from build123d import *

# Parameters (mm, degrees)
F4_DEPTH    = 13
F5_R        = 7
F6_DEPTH    = 15
F7_R        = 14.5
F8_DEPTH    = 1.6
F9_S5_R     = 14.5
F9_T6_DEPTH = 29
F10_SIZE    = 5


# Not quite as in the source:
# - a fillet or chamfer that OpenCascade refuses, or shapes differently, is made with other operations: its cross-section is extruded or revolved along the edge and cut away or added
# - a feature names something its author has since deleted; it is built from what else it names


with BuildPart() as f2:
    # F0 (on Front) → F2 (revolve)
    with BuildSketch(Plane.XZ):
        Polygon((17.6, 24.4003517207), (0, 24.4003517207), (0, 23.0003517207), (14, 23.0003517207), (33.795146799, -22.8053483963), (43.2849223453, -22.5459427606), (43.2849223453, -21.1459427606), (37.9849223453, -21.1459427606), align=None)
    revolve(axis=Axis((0, 0, 12.0206931606), (0, 0, -1)))

    # F3 (on face) → F4 (join)
    with BuildSketch(Plane.XY.offset(24.4003517207)):
        Polygon((-11.9566419536, 1.0191727989), (-6.8609505115, -9.8451692763), (5.0956914421, -10.8643420752), (11.9566419536, -1.0191727989), (6.8609505115, 9.8451692763), (-5.0956914421, 10.8643420752), align=None)
    extrude(amount=F4_DEPTH)

    # F5 (on face) → F6 (cut)
    with BuildSketch(Plane.XY.offset(37.4003517207)):
        Circle(F5_R)
    extrude(amount=-F6_DEPTH, mode=Mode.SUBTRACT)

    # F7 (on face) → F8 (join)
    with BuildSketch(Plane.XY.offset(24.4003517207)):
        Circle(F7_R)
    extrude(amount=F8_DEPTH)

    # F9: chamfer of 4 on 1 edges, made by hand


with BuildPart() as f9_tool2:
    # F9_s3 → F9_t4 (revolve)
    with BuildSketch(Plane.XZ):
        Polygon((19.2340619114, 20.749346151), (13.6, 24.4003517207), (17.6, 24.4003517207), align=None)
    revolve(axis=Axis((0, 0, 24.4003517207), (0, 0, -1)))

    # F9_s5 → F9_t6 (cut, symmetric)
    with BuildSketch(Plane.XY.offset(22.6)):
        Circle(F9_S5_R)
    extrude(amount=F9_T6_DEPTH, both=True, mode=Mode.SUBTRACT)


with BuildPart() as f2_1:
    add(f2.part)

    # F9_t1: cut F9_tool2
    add(f9_tool2.part, mode=Mode.SUBTRACT)

    # F10
    f10_edges = [f2_1.edges().sort_by_distance(p)[0] for p in [
        (-37.984922, 0, -21.145943),
    ]]
    chamfer(f10_edges, length=F10_SIZE)


solid = f2_1.part
Work out the finished part from the listing and answer in its coordinate system (mm). A direction names the side the tool comes from. Give positions to 0.01 mm unless a question says otherwise; leave off trailing zeros. Loops run counter-clockwise (first coordinate to the right, second up) from the corner with the lowest first, then second, coordinate; pieces in that order, holes last. Notation, with made-up numbers: (-31, 0.25) -> (12, 0.25) arc R28 ccw to (12, 25.25) -> close; hole circle Ø3 at (43, 62). An arc over 180 degrees is marked (long way). Use a Markdown table: item, result. Add a question column.
1. Determine the mould class of faces 5 (the flat face through (0, 0, 24.4)), 6 (the flat face through (-1, -11, 26)), 7 (the flat face through (-0.966, -10.348, 31.621)), 8 (the cylindrical face through (6.691, -12.864, 24.924)) for opening direction Y: released by +Y, released by -Y, zero draft, split by the parting line, or undercut.
2. Flat-ended cylindrical pins translate along their axes: pin 1 Ø4 at (x, y) = (8.5, -13) entering from -Z; pin 2 Ø1 at (y, z) = (4.5, -12.5) entering from +X; pin 3 Ø14 at (x, y) = (-7, 2) entering from -Z. Find the tip coordinate at first contact, or state that the pin passes through.
3. Section B-B on z = 29.5 is taken. Determine the outline of the cut face in (x, y).
4. Section C-C on z = 5.5 is taken. Determine the outline of the cut face in (x, y).
5. Section D-D on z = -12 is taken. Determine the outline of the cut face in (x, y), and give its area (3 significant figures).
6. For faces 1 (the flat face through (0, 0, 26)), 2 (the flat face through (8.48, -6.01, 31.62)), 3 (the flat face through (9.444, 4.337, 31.621)), 4 (the cylindrical face through (6.466, -2.681, 23.71)), determine the directions among +Z, -Z, +X, -X, +Y, -Y from which every point of the face is accessible in a straight line to the end or side of a thin tool.
7. Find the intervals of material crossed by probe 1 along Y at (x, z) = (0, 24.15); probe 2 along X at (y, z) = (3, 34); probe 3 along Y at (x, z) = (-9, 2), in increasing order.
Results below:
| question | item | result |
|---|---|---|
| 1 | face 5 | undercut |
| 1 | face 6 | zero draft |
| 1 | face 7 | released by -Y |
| 1 | face 8 | split by the parting line |
| 2 | pin 1 | stops at z = 14.83 |
| 2 | pin 2 | stops at x = 34.05 |
| 2 | pin 3 | stops at z = 22.35 |
| 3 | outline | (-11.96, 1.02) -> (-6.86, -9.85) -> (5.1, -10.86) -> (11.96, -1.02) -> (6.86, 9.85) -> (-5.1, 10.86) -> close; hole circle Ø14 at (0, 0) |
| 4 | outline | circle Ø52.12 at (0, 0); hole circle Ø43.13 at (0, 0) |
| 5 | outline | circle Ø67.78 at (0, 0); hole circle Ø58.25 at (0, 0) |
| 5 | area | 944 mm^2 |
| 6 | face 1 | +Z |
| 6 | face 2 | +Z, +X, -Y |
| 6 | face 3 | +Z, +X, +Y |
| 6 | face 4 | -Z |
| 7 | probe 1 | y = -14.5 to -7, 7 to 14.5 |
| 7 | probe 2 | x = -10.58 to -6.32, 6.32 to 10.07 |
| 7 | probe 3 | y = -26.12 to -21.25, 21.25 to 26.12 |
